Part model, mm, in its own coordinate system. Round coordinates to 2 decimals unless told otherwise and drop trailing zeros. Write each loop counter-clockwise with the first axis right and the second up, starting at its lowest first coordinate (ties: lowest second). Pieces come first, ordered by that corner, then holes.
from build123d import *

# Parameters (mm, degrees)
SKETCH1_W           = 101.6
SKETCH1_H           = 22.225
SKETCH1_R           = 3.2639
BOSS_EXTRUDE1_DEPTH = 2.38125


with BuildPart() as part:
    # Sketch1 → Boss-Extrude1 (new, symmetric)
    with BuildSketch(Plane.XY):
        with Locations((50.8, 11.1125)):
            Rectangle(SKETCH1_W, SKETCH1_H)
        with Locations(Location((12.7, 11.1125, 0), (0, 0, 180))):
            Circle(SKETCH1_R, mode=Mode.SUBTRACT)
        with Locations(Location((38.1, 11.1125, 0), (0, 0, 180))):
            Circle(SKETCH1_R, mode=Mode.SUBTRACT)
        with Locations(Location((63.5, 11.1125, 0), (0, 0, 180))):
            Circle(SKETCH1_R, mode=Mode.SUBTRACT)
        with Locations(Location((88.9, 11.1125, 0), (0, 0, 180))):
            Circle(SKETCH1_R, mode=Mode.SUBTRACT)
    extrude(amount=BOSS_EXTRUDE1_DEPTH, both=True)


solid = part.part
Q1. Wall check: line 1 (Y direction, x = 88.9, z = 0.6) (3 decimals); line 2 (X direction, y = 8.25, z = 1.2); line 3 (X direction, y = 9.25, z = 1.45). Give the ranges that are in metal, low to high.
Q2. Saw through at C-C, the plane y = 9. Write the cut outline in (x, z), and give its area (3 significant figures).
Q3. Drop a flat-ended pin along its axis: P1, Ø4, axis at x = 12.7, y = 11.11, coming from the +Z side. Give the stop position or say it passes through.
Q4. Saw through at B-B, the plane z = 0.15. Write the cut outline in (x, y) (1 decimal).
Q5. Saw through at A-A, the plane x = 12.7. Write the cut outline in (y, z) (3 decimals), and give its area (3 significant figures).
Q6. Saw through at D-D, the plane x = 90. Write the cut outline in (y, z) (3 decimals).
Q7. Two-plate mould, pull along Y, no slides. Class faces 1 (the cylindrical face through (15.29, 13.1, -0.03)), 2 (the flat face through (101.6, 11, 0)), 3 (the flat face through (50, 22.225, 0)): released by +Y, released by -Y, zero draft, split by the parting line, or undercut.
Computed:
1. line 1: y = 0 to 7.849, 14.376 to 22.225
1. line 2: x = 0 to 11.13, 14.27 to 36.53, 39.67 to 61.93, 65.07 to 87.33, 90.47 to 101.6
1. line 3: x = 0 to 10.02, 15.38 to 35.42, 40.78 to 60.82, 66.18 to 86.22, 91.58 to 101.6
2. outline: (0, -2.38) - (10.21, -2.38) - (10.21, 2.38) - (0, 2.38) - close; (15.19, -2.38) - (35.61, -2.38) - (35.61, 2.38) - (15.19, 2.38) - close; (40.59, -2.38) - (61.01, -2.38) - (61.01, 2.38) - (40.59, 2.38) - close; (65.99, -2.38) - (86.41, -2.38) - (86.41, 2.38) - (65.99, 2.38) - close; (91.39, -2.38) - (101.6, -2.38) - (101.6, 2.38) - (91.39, 2.38) - close
2. area: 389 mm2
3. P1: passes through
4. outline: (0, 0) - (101.6, 0) - (101.6, 22.2) - (0, 22.2) - close; hole circle Ø6.5 at (12.7, 11.1); hole circle Ø6.5 at (38.1, 11.1); hole circle Ø6.5 at (63.5, 11.1); hole circle Ø6.5 at (88.9, 11.1)
5. outline: (0, -2.381) - (7.849, -2.381) - (7.849, 2.381) - (0, 2.381) - close; (14.376, -2.381) - (22.225, -2.381) - (22.225, 2.381) - (14.376, 2.381) - close
5. area: 74.8 mm2
6. outline: (0, -2.381) - (8.04, -2.381) - (8.04, 2.381) - (0, 2.381) - close; (14.185, -2.381) - (22.225, -2.381) - (22.225, 2.381) - (14.185, 2.381) - close
7. face 1: undercut
7. face 2: zero draft
7. face 3: released by +Y
